Design review of the part built by this model. Coordinates are the model's own, in mm. Face numbers are marked on the shaded views. Coordinates: 2 decimals unless noted, no trailing zeros. Write each loop counter-clockwise with the first axis right and the second up, starting at its lowest first coordinate (ties: lowest second). Pieces come first, ordered by that corner, then holes.
Q1. Add section D-D, the plane x = 32. Give the boundary of the cut face in (y, z).
Q2. Add section A-A, the plane y = 29.5. Give the boundary of the cut face in (x, z).
Q3. The part is to be moulded in two halves that separate along Y. For the marked faces 1, 2 and 3, say which applies: +Y half, -Y half, draft (parallel to the pull), parting line (faces both ways), or undercut.
Q4. To check wall thickness, follow probe 1 along Z at (x, y) = (25.5, 8); probe 2 along X at (y, z) = (21, 18); probe 3 along Z at (x, y) = (-30, 14.5). State the ranges of each line that lie inside material, in increasing order.
Q5. Clearance check with flat-ended pins moving along their axes: pin 1 Ø12 at (x, y) = (27.5, 35) entering from +Z; pin 2 Ø2 at (x, y) = (-27.5, 25) entering from +Z; pin 3 Ø10 at (y, z) = (9.5, 36) entering from +X. State where each tip first meets the part, or that it passes through.
Q6. Add section B-B, the plane y = 47. Give the boundary of the cut face in (x, z).
Q7. Add section C-C, the plane y = 38. Give the boundary of the cut face in (x, z), plus the area to 3 significant figures.
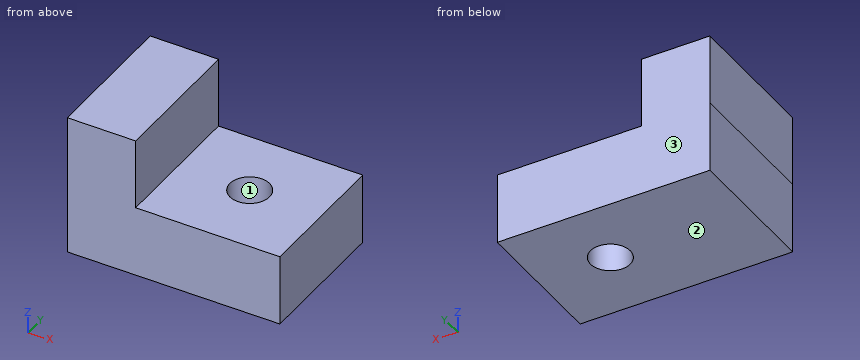
from build123d import *

# Parameters (mm, degrees)
F1_DEPTH = 60
F2_W     = 29.0517922733
F2_H     = 60
F3_DEPTH = 30
F4_R     = 8.4402265008
F5_DEPTH = 49


with BuildPart() as f1:
    # F0 (on Front) → F1 (new body)
    with BuildSketch(Plane.XZ):
        Polygon((51.5215955675, 16.4024308324), (-38.782004267, 16.4853166789), (-38.782004267, -13.7799708173), (51.5215955675, -13.7799708173), align=None)
    extrude(amount=-F1_DEPTH)

    # F2 (on face) → F3 (join)
    with BuildSketch(Plane(origin=(0.0150984883, 0, 16.4497064628), x_dir=(0.9999995788, 0, -0.0009178572), z_dir=(0.0009178572, 0, 0.9999995788))):
        with Locations((-24.2712229612, 30)):
            Rectangle(F2_W, F2_H)
    extrude(amount=F3_DEPTH)

    # F4 (on face) → F5 (cut)
    with BuildSketch(Plane(origin=(0.0150984883, 0, 16.4497064628), x_dir=(0.9999995788, 0, -0.0009178572), z_dir=(0.0009178572, 0, 0.9999995788))):
        with Locations((20.6399001181, 30.7776089758)):
            Circle(F4_R)
    extrude(amount=-F5_DEPTH, mode=Mode.SUBTRACT)


solid = f1.part
Here are the results:
1. outline: (0, -13.78) - (60, -13.78) - (60, 16.42) - (0, 16.42) - close
2. outline: (-38.78, -13.78) - (12.28, -13.78) - (12.31, 16.44) - (-9.73, 16.46) - (-9.7, 46.46) - (-38.75, 46.49) - (-38.78, 16.49) - close; (28.97, -13.78) - (51.52, -13.78) - (51.52, 16.4) - (29, 16.42) - close
3. face 1: undercut
3. face 2: draft
3. face 3: +Y half
4. probe 1: z = -13.78 to 16.43
4. probe 2: x = -38.78 to -9.73
4. probe 3: z = -13.78 to 46.48
5. pin 1: stops at z = 16.43
5. pin 2: stops at z = 46.48
5. pin 3: stops at x = -9.71
6. outline: (-38.78, -13.78) - (51.52, -13.78) - (51.52, 16.4) - (-9.73, 16.46) - (-9.7, 46.46) - (-38.75, 46.49) - (-38.78, 16.49) - close
7. outline: (-38.78, -13.78) - (16.26, -13.78) - (16.29, 16.43) - (-9.73, 16.46) - (-9.7, 46.46) - (-38.75, 46.49) - (-38.78, 16.49) - close; (24.99, -13.78) - (51.52, -13.78) - (51.52, 16.4) - (25.02, 16.43) - close
7. area: 3,340 mm2
